from build123d import *

# Parameters (mm, degrees)
SKETCH1_W                  = 40
SKETCH1_H                  = 28.5
BOSS_EXTRUDE1_DEPTH        = 5
M2_TAPPED_HOLE1_AT_2_COUNT = 2
M2_TAPPED_HOLE1_AT_2_PITCH = 20


with BuildPart() as part:
    # Sketch1 → Boss-Extrude1 (new body)
    with BuildSketch(Plane.XY):
        Rectangle(SKETCH1_W, SKETCH1_H)
    extrude(amount=BOSS_EXTRUDE1_DEPTH)

    # Sketch4 → M2 Tapped Hole1 (revolve, cut)
    with BuildSketch(Plane(origin=(-10, 14.25, 2.5), x_dir=(0, 0, 1), z_dir=(1, 0, 0))):
        Polygon((0, 0), (0, 5.480688495), (0.8, 5), (0.8, 0), align=None)
    m2_tapped_hole1 = revolve(axis=Axis((-10, 20.6, 2.5), (0, -1, 0)), mode=Mode.SUBTRACT)

    # M2 Tapped Hole1 at 2: M2 Tapped Hole1 ×2
    with Locations(*[(i * M2_TAPPED_HOLE1_AT_2_PITCH, 0, 0) for i in range(1, M2_TAPPED_HOLE1_AT_2_COUNT)]):
        add(m2_tapped_hole1, mode=Mode.SUBTRACT)

    # Mirror1: M2 Tapped Hole1 across plane
    add(m2_tapped_hole1.mirror(Plane.ZX), mode=Mode.SUBTRACT)

    # Mirror1 copy 1 sketch → Mirror1 copy 1 (revolve, cut)
    with BuildSketch(Plane(origin=(10, -14.25, 2.5), x_dir=(0, 0, 1), z_dir=(1, 0, 0))):
        Polygon((0, 0), (0, -5.480688495), (0.8, -5), (0.8, 0), align=None)
    revolve(axis=Axis((10, -20.6, 2.5), (0, -1, 0)), mode=Mode.SUBTRACT)


solid = part.part
Can you work these out from the model? Positions are in its coordinate system, mm. A direction names the side the tool comes from. Round coordinates to 2 decimals unless told otherwise and drop trailing zeros. Order: outer loops, then holes, each group sorted by start corner. A loop starts at its lowest first (then second) coordinate and runs counter-clockwise, first axis right, second up. Notation, with made-up numbers: M 31.25,-29.5 L 74.25,-29.5 A21 cw 74.25,7.5 Z; hole C -32,-13.75 d7. An arc over 180 degrees is marked long. Use a Markdown table: item, result.
1) Imagine slicing it at A-A (y = 10.25). List the corners of the cut face in (x, z) for me, then the cut area to 3 significant figures.
Geometry says:
| item | result |
|---|---|
| outline | M -20,0 L 20,0 L 20,5 L -20,5 Z; hole C -10,2.5 d1.6; hole C 10,2.5 d1.6 |
| area | 196 mm² |
2) If I drill on line 1 along X through (y, z) = (-10.4, 2.5); line 2 along Z through (x, y) = (-10, -12.05); line 3 along X through (y, z) = (9.5, 2.2), over which ranges is the centre line in solid material (lowest first)?
Geometry says:
| item | result |
|---|---|
| line 1 | x = -20 to -10.8, -9.2 to 9.2, 10.8 to 20 |
| line 2 | z = 0 to 1.7, 3.3 to 5 |
| line 3 | x = -20 to -10.74, -9.26 to 9.26, 10.74 to 20 |
3) On a 3-axis mill with a long thin cutter (end or side, diameter ignored), from which of +Z, -Z, +X, -X, +Y, -Y can I reach the whole of each face in a straight line? I mean faces 1 (the face through (-10.793, 11.785, 2.396)), 2 (the face through (-10.793, -11.785, 2.396)), 3 (the face through (-20, 0, 2)). Say none if no direction works.
Geometry says:
| item | result |
|---|---|
| face 1 | +Y |
| face 2 | -Y |
| face 3 | +Z, -Z, -X, +Y, -Y |
4) If we mould it in two halves opening along Z, with no side actions, what happens to faces 4 (the face through (0, 0, 0)), 5 (the face through (9.883, -8.853, 2.575)), 6 (the face through (20, 0, 2))? For each: +Z half, -Z half, draft (parallel to the pull), parting line (faces both ways), or undercut.
Geometry says:
| item | result |
|---|---|
| face 4 | -Z half |
| face 5 | undercut |
| face 6 | draft |
5) I'm going to push flat-ended pins straight in: P1, Ø1.4, axis at x = 10, z = 2.5, coming from the -Y side; P2, Ø1.4, axis at x = -10, z = 2.5, coming from the +Y side. Where does each tip first touch, or does it pass through?
Geometry says:
| item | result |
|---|---|
| P1 | stops at y = -9.19 |
| P2 | stops at y = 9.19 |
